Design review of the part built by this model. Coordinates are the model's own, in mm. A direction names the side the tool comes from. Round coordinates to 2 decimals unless told otherwise and drop trailing zeros. Order: outer loops, then holes, each group sorted by start corner. A loop starts at its lowest first (then second) coordinate and runs counter-clockwise, first axis right, second up. Notation, with made-up numbers: (68, 50.5) - (104, 50.5) arc R22 ccw to (104, 56.5) - close; hole circle Ø6 at (67.5, 82.25). An arc over 180 degrees is marked (long way). Answer as a JSON object with one key per item and string values. Group by question number.
from build123d import *

# Parameters (mm, degrees)
SKETCH1_R           = 4.029111805
BOSS_EXTRUDE3_DEPTH = 9.652
SKETCH3_R           = 7.14375
SKETCH3_R_2         = 4.029111805
BOSS_EXTRUDE4_DEPTH = 2.032
FILLET2_R           = 2.54
SKETCH4_R           = 4.655068421
CUT_EXTRUDE1_DEPTH  = 0.762


with BuildPart() as part:
    # Sketch1 → Boss-Extrude3 (new body)
    with BuildSketch(Plane(origin=(0, 0, 0), x_dir=(1, 0, 0), z_dir=(0, 1, 0))):
        Polygon((-7.14375, 4.124445986), (-7.14375, 0), (-7.14375, -4.124445986), (0, -8.248891971), (3.571875, -6.186668978), (7.14375, -4.124445986), (7.14375, 0), (7.14375, 4.124445986), (0, 8.248891971), (-3.571875, 6.186668978), align=None)
        with Locations(Location((0, 0, 0), (0, 0, 270))):
            Circle(SKETCH1_R, mode=Mode.SUBTRACT)
    extrude(amount=BOSS_EXTRUDE3_DEPTH)

    # Sketch3 → Boss-Extrude4 (add)
    with BuildSketch(Plane(origin=(0, 9.652, 0), x_dir=(1, 0, 0), z_dir=(0, 1, 0))):
        with Locations(Location((0, 0, 0), (0, 0, 60))):
            Circle(SKETCH3_R)
        with Locations(Location((0, 0, 0), (0, 0, 270))):
            Circle(SKETCH3_R_2, mode=Mode.SUBTRACT)
    extrude(amount=BOSS_EXTRUDE4_DEPTH)

    # Fillet2
    # the kernel refuses this fillet: 2.54 mm, written as the material it takes off along each edge
    with BuildSketch(Plane(origin=(0, 11.684, 0), x_dir=(0.5000000000000001, 0, -0.8660254037844386), z_dir=(0.8660254037844386, 0, 0.5000000000000001))) as fillet2_piece_1:
        with BuildLine():
            CenterArc((4.655068421, -2.54), FILLET2_R, 11.536959033, 78.463040967)
            Line((7.14375, -2.032), (7.193523632, -2.02184))
            ThreePointArc((7.193523632, -2.02184), (7.19455, -1.016), (7.19455, 0))
            Line((7.19455, 0), (7.14375, 0.0508))
            Line((7.14375, 0.0508), (4.655068421, 0.0508))
            Line((4.655068421, 0.0508), (4.655068421, 0))
        make_face()
    revolve(axis=Axis((0, 11.684, 0), (0, 1, 0)), mode=Mode.SUBTRACT)

    # Sketch4 → Cut-Extrude1 (cut)
    with BuildSketch(Plane(origin=(0, 11.684, 0), x_dir=(1, 0, 0), z_dir=(0, 1, 0))):
        with Locations(Location((0, 0, 0), (0, 0, 270))):
            Circle(SKETCH4_R)
    extrude(amount=-CUT_EXTRUDE1_DEPTH, mode=Mode.SUBTRACT)


solid = part.part
1. Mouldability with a two-part tool opening along X and no side actions: class faces 1 (the flat face through (3.62, 4.76, -6.16)), 2 (the cylindrical face through (-2.45, 5.38, -3.2)), 3 (the flat face through (-7.144, 5, 0)) as pulls with the +X half, pulls with the -X half, needs draft (parallel to the pull), parting line crosses it, or undercut.
2. Take a section at A-A, the plane y = 3. Give the boundary of the cut face in (x, z).
3. To check wall thickness, follow line 1 (X direction, y = 1, z = 0); line 2 (Z direction, x = 0, y = 11.45); line 3 (Z direction, x = -1.5, y = 7.75). State the ranges of each line that lie inside material, in increasing order. Write a range as from..to.
4. Tool access review of faces 4 (the flat face through (-6.4, 9.652, 3.8)), 5 (the flat face through (-6.4, 9.652, -3.6)), 6 (the flat face through (6.4, 9.652, -3.6)): name each direction out of +Z, -Z, +X, -X, +Y, -Y from which nothing blocks a thin tool from reaching the whole face with its end or side.
5. Clearance check with flat-ended pins moving along their axes: P1, Ø6.5, axis at x = 0, z = 0, coming from the +Y side; P2, Ø1, axis at x = -0.5, y = 10.5, coming from the +Z side; P3, Ø3, axis at x = -5.5, z = 2, coming from the +Y side; P4, Ø4, axis at x = -6, z = -4, coming from the +Y side. State where each tip first meets the part, or that it passes through.
Response values:
{
 "1": {"face 1": "pulls with the +X half", "face 2": "undercut", "face 3": "pulls with the -X half"},
 "2": {"outline": "(-7.14, -4.12) - (0, -8.25) - (7.14, -4.12) - (7.14, 4.12) - (0, 8.25) - (-7.14, 4.12) - close; hole circle Ø8.06 at (0, 0)"},
 "3": {"line 1": "-7.14..-4.03, 4.03..7.14", "line 2": "-5.72..-4.66, 4.66..5.72", "line 3": "-7.38..-3.74, 3.74..7.38"},
 "4": {"face 4": "+Z, -X, +Y", "face 5": "-Z, -X, +Y", "face 6": "-Z, +X, +Y"},
 "5": {"P1": "through", "P2": "z = 7.03", "P3": "y = 11.68", "P4": "y = 11.62"}
}
